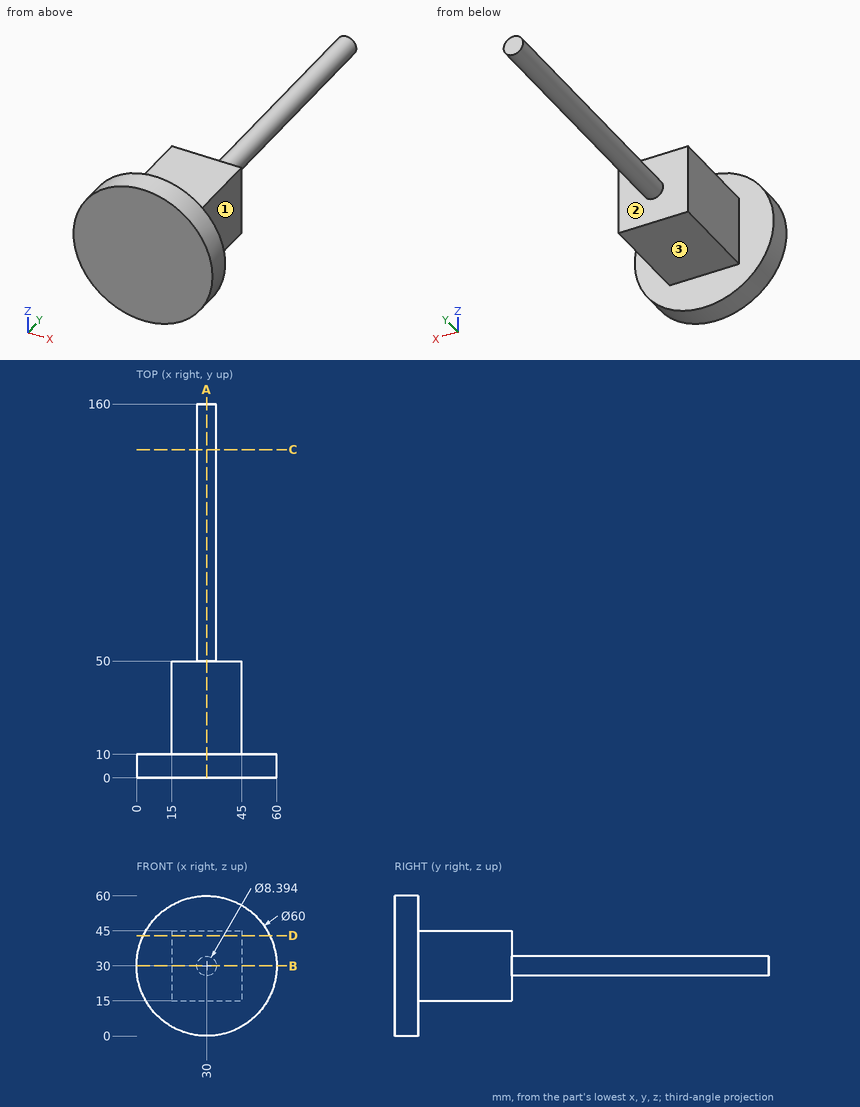
Verification items for this drawing (mm, ordinates from the low corner). A direction names the side the tool comes from. Coordinates: 2 decimals unless noted, no trailing zeros. Write each loop counter-clockwise with the first axis right and the second up, starting at its lowest first coordinate (ties: lowest second). Pieces come first, ordered by that corner, then holes. Notation, with made-up numbers: M 60.5,-20 L 104.5,-20 A36 ccw 104.5,15 Z; hole C 32,45 d4. An arc over 180 degrees is marked long. Answer as CSV lines item,"result".
Q1. Set-up check for the marked faces 1, 2 and 3: record each of +Z, -Z, +X, -X, +Y, -Y from which the full face is reachable in a straight line by a thin tool's end or side.
Check result:
face 1,"+Z, -Z, +X, +Y"
face 2,"+Y"
face 3,"-Z, +X, -X, +Y"
Q2. Go/stop test with flat-tipped pins: pin 1 (15 mm diameter, centred on y = 29.5, z = 30, fed in from +X); pin 2 (12 mm diameter, centred on y = 73, z = 23, fed in from +X); pin 3 (15 mm diameter, centred on x = 26.5, y = 35, fed in from +Z). Record where each tip stops, or that it passes through.
Check result:
pin 1,"x = 45"
pin 2,"x = 34.08"
pin 3,"z = 45"
Q3. Cross-section at A-A (x = 30). Record the boundary of the cut face in (y, z).
Check result:
outline,"M 0,0 L 10,0 L 10,15 L 50,15 L 50,25.8 L 160,25.8 L 160,34.2 L 50,34.2 L 50,45 L 10,45 L 10,60 L 0,60 Z"
Q4. Cross-section at C-C (y = 140.5). Record the boundary of the cut face in (x, z).
Check result:
outline,"C 30,30 d8.39"
Q5. Material ranges on probe 1 along Y at (x, z) = (40, 26); probe 2 along Y at (x, z) = (28.5, 47.5); probe 3 along Z at (x, y) = (30, 19), recorded low to high. Write a range as from..to.
Check result:
probe 1,"0..50"
probe 2,"0..10"
probe 3,"15..45"
Q6. Cross-section at D-D (z = 43). Record the boundary of the cut face in (x, y).
Check result:
outline,"M 2.96,0 L 57.04,0 L 57.04,10 L 45,10 L 45,50 L 15,50 L 15,10 L 2.96,10 Z"
Q7. Cross-section at B-B (z = 30). Record the boundary of the cut face in (x, y).
Check result:
outline,"M 0,0 L 60,0 L 60,10 L 45,10 L 45,50 L 34.2,50 L 34.2,160 L 25.8,160 L 25.8,50 L 15,50 L 15,10 L 0,10 Z"
